```python
from build123d import *

# Parameters (mm, degrees)
SKIZZE4_R                            = 3
AUFSATZ_LINEAR_AUSTRAGEN1_DEPTH      = 4
AUFSATZ_LINEAR_AUSTRAGEN1_DEPTH_BACK = 4


with BuildPart() as part:
    # Skizze4 → Aufsatz-Linear austragen1 (new body, two sides)
    with BuildSketch(Plane.XY) as aufsatz_linear_austragen1_sk:
        Polygon((-10, 610), (-10, 570), (10, 570), (10, 610), (10, 618), (-10, 618), align=None)
        with Locations((0, 610)):
            Circle(SKIZZE4_R, mode=Mode.SUBTRACT)
    extrude(amount=AUFSATZ_LINEAR_AUSTRAGEN1_DEPTH)
    extrude(aufsatz_linear_austragen1_sk.sketch, amount=-AUFSATZ_LINEAR_AUSTRAGEN1_DEPTH_BACK)


solid = part.part
```
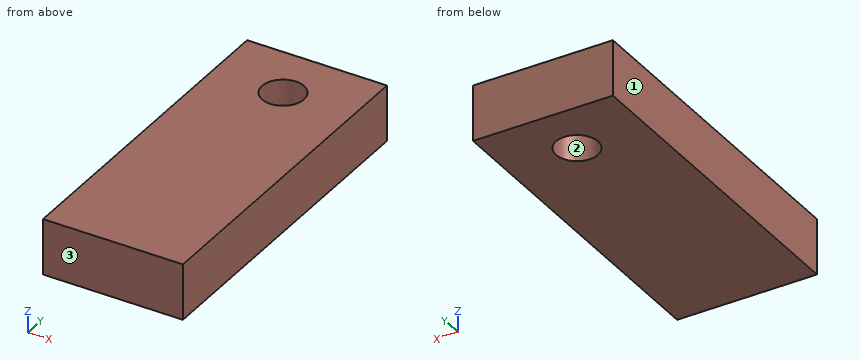
CAD build for the part. Positions are in the model's coordinates, mm. Face numbers are marked on the shaded views. Coordinates: 2 decimals unless noted, no trailing zeros. Order: outer loops, then holes, each group sorted by start corner. A loop starts at its lowest first (then second) coordinate and runs counter-clockwise, first axis right, second up. Notation, with made-up numbers: (88.5, 74.25) -> (141.5, 74.25) arc R17 ccw to (141.5, 93.25) -> close; hole circle Ø11 at (7.5, -5.75). An arc over 180 degrees is marked (long way). Use one line per item in the form item = value. Start each with the question number.
1) Band-saw the part on B-B on y = 610. Give the cut face in (x, z), then the cut area to 3 significant figures.
2) Band-saw the part on C-C on z = -1. Give the cut face in (x, y).
3) Drill centre lines: L1, parallel to Y at x = 0, z = 0.25; L2, parallel to X at y = 610, z = -2.25; L3, parallel to Y at x = 1.25, z = -2.75. Where is each one in solid material? Low to high. Write a range as [from, to].
4) Pull direction Y, two halves, no side cores. Call the marked faces 1, 2 and 3: +Y half, -Y half, draft (parallel to the pull), parting line (faces both ways), or undercut.
5) Band-saw the part on A-A on x = 0. Give the cut face in (y, z), then the cut area to 3 significant figures.
Entries:
q1.outline = (-10, -4) -> (-3, -4) -> (-3, 4) -> (-10, 4) -> close; (3, -4) -> (10, -4) -> (10, 4) -> (3, 4) -> close
q1.area = 112 mm2
q2.outline = (-10, 570) -> (10, 570) -> (10, 618) -> (-10, 618) -> close; hole circle Ø6 at (0, 610)
q3.L1 = [570, 607], [613, 618]
q3.L2 = [-10, -3], [3, 10]
q3.L3 = [570, 607.27], [612.73, 618]
q4.face_1 = draft
q4.face_2 = undercut
q4.face_3 = -Y half
q5.outline = (570, -4) -> (607, -4) -> (607, 4) -> (570, 4) -> close; (613, -4) -> (618, -4) -> (618, 4) -> (613, 4) -> close
q5.area = 336 mm2
